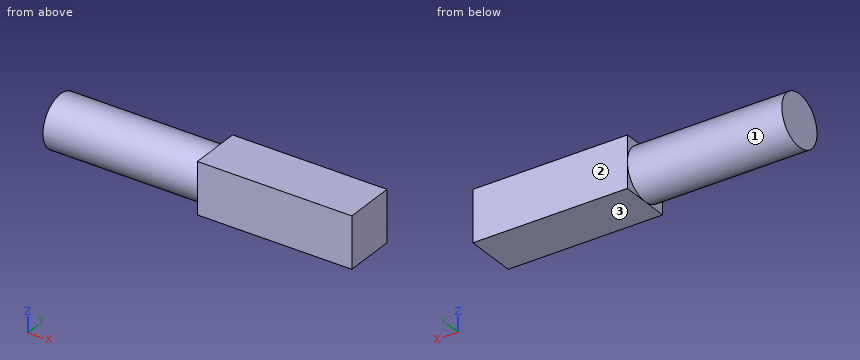
from build123d import *

# Parameters (mm, degrees)
F0_R     = 2.5
F1_DEPTH = 15
F2_W     = 5
F2_H     = 5
F3_DEPTH = 15


with BuildPart() as f1:
    # F0 (on Right) → F1 (new body)
    with BuildSketch(Plane.YZ):
        Circle(F0_R)
    extrude(amount=F1_DEPTH)

    # F2 (on face) → F3 (join)
    with BuildSketch(Plane.YZ.offset(15)):
        Rectangle(F2_W, F2_H)
    extrude(amount=F3_DEPTH)


solid = f1.part
Here's how the part is built. I have some questions about the finished solid (model axes, mm). Face numbers are marked on the shaded views. Coordinates: 2 decimals unless noted, no trailing zeros. Write each loop counter-clockwise with the first axis right and the second up, starting at its lowest first coordinate (ties: lowest second). Pieces come first, ordered by that corner, then holes.
Item 1: I want a section at B-B on y = 1.75. Write out the boundary of the cut face in (x, z), and give its area (3 significant figures).
Item 2: I want a section at C-C on x = 5. Write out the boundary of the cut face in (y, z), and give its area (3 significant figures).
Item 3: I want a section at A-A on z = -0.7. Write out the boundary of the cut face in (x, y).
Item 4: If we mould it in two halves opening along Y, with no side actions, what happens to the marked faces 1, 2 and 3? For each: +Y half, -Y half, draft (parallel to the pull), parting line (faces both ways), or undercut.
Item 5: If I drill on line 1 (X direction, y = 2.15, z = -1.45); line 2 (Z direction, x = 5.25, y = -2.3); line 3 (Y direction, x = 4.75, z = -0.65), over which ranges is the centre line in solid material (lowest first)?
Findings below:
1. outline: (0, -1.79) - (15, -1.79) - (15, -2.5) - (30, -2.5) - (30, 2.5) - (15, 2.5) - (15, 1.79) - (0, 1.79) - close
1. area: 129 mm2
2. outline: circle Ø5 at (0, 0)
2. area: 19.6 mm2
3. outline: (0, -2.4) - (15, -2.4) - (15, -2.5) - (30, -2.5) - (30, 2.5) - (15, 2.5) - (15, 2.4) - (0, 2.4) - close
4. face 1: parting line
4. face 2: +Y half
4. face 3: draft
5. line 1: x = 15 to 30
5. line 2: z = -0.98 to 0.98
5. line 3: y = -2.41 to 2.41
